The drawing under review shows one solid part. Ordinate dimensions are in mm from its lowest x, y, z. A direction names the side the tool comes from. Round coordinates to 2 decimals unless told otherwise and drop trailing zeros. Loops run counter-clockwise (first coordinate to the right, second up) from the corner with the lowest first, then second, coordinate; pieces in that order, holes last. Notation, with made-up numbers: (52.25, 3.5) - (100.25, 3.5) arc R26 cw to (100.25, 19.5) - close; hole circle Ø9 at (-16, 55). An arc over 180 degrees is marked (long way). Answer as CSV lines item,"result".
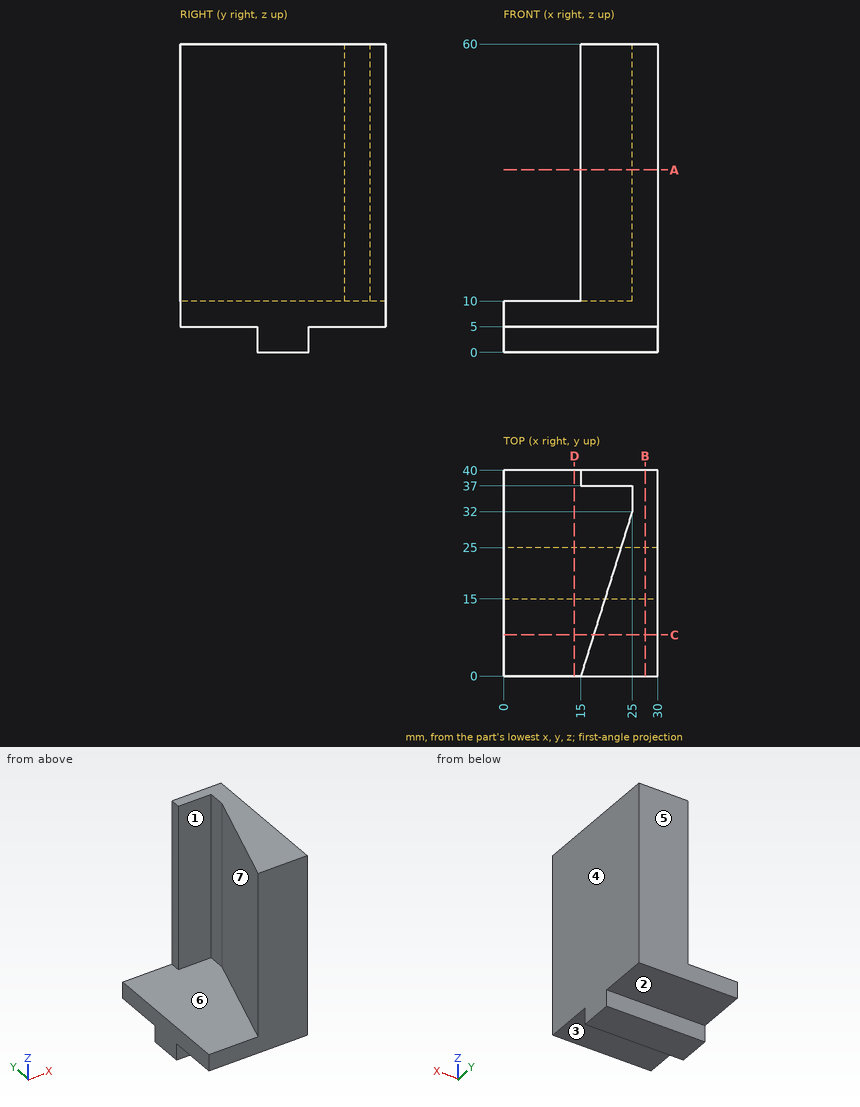
1. Take a section at D-D (x = 13.75). State the section outline as (y, z) points.
Numbers:
outline,"(0, 5) - (15, 5) - (15, 0) - (25, 0) - (25, 5) - (40, 5) - (40, 10) - (0, 10) - close"
2. Tool access review of the marked faces 1, 2 and 3: name each direction out of +Z, -Z, +X, -X, +Y, -Y from which nothing blocks a thin tool from reaching the whole face with its end or side.
Numbers:
face 1,"+Z, -X"
face 2,"-Z, +X, -X, +Y"
face 3,"-Z, +X, -X, -Y"
3. Wall thickness on probe 1 along Z at (x, y) = (9.25, 13); probe 2 along Z at (x, y) = (7.75, 24.5); probe 3 along Y at (x, z) = (4.75, 3.5): over which ranges is each line inside the solid? List them lowest first.
Numbers:
probe 1,"z = 5 to 10"
probe 2,"z = 0 to 10"
probe 3,"y = 15 to 25"
4. Draft analysis for pull direction Y (two halves, no side actions). For the marked faces 4, 5, 6 and 7, state which applies: +Y half, -Y half, draft (parallel to the pull), parting line (faces both ways), or undercut.
Numbers:
face 4,"draft"
face 5,"+Y half"
face 6,"undercut"
face 7,"undercut"
5. Take a section at C-C (y = 8). State the section outline as (x, z) points, plus the area to 3 significant figures.
Numbers:
outline,"(0, 5) - (30, 5) - (30, 60) - (17.5, 60) - (17.5, 10) - (0, 10) - close"
area,"775 mm²"
6. Clearance check with flat-ended pins moving along their axes: pin 1 (1 mm diameter, centred on x = 6, y = 33.5, fed in from +Z); pin 2 (1.5 mm diameter, centred on y = 24, z = 36.5, fed in from -X); pin 3 (5.5 mm diameter, centred on y = 35.5, z = 24, fed in from -X). State where each tip first meets the part, or that it passes through.
Numbers:
pin 1,"stops at z = 10"
pin 2,"stops at x = 22.27"
pin 3,"stops at x = 15"
7. Take a section at A-A (z = 35.5). State the section outline as (x, y) points.
Numbers:
outline,"(15, 0) - (30, 0) - (30, 40) - (15, 40) - (15, 37) - (25, 37) - (25, 32) - close"
8. Take a section at B-B (x = 27.5). State the section outline as (y, z) points.
Numbers:
outline,"(0, 5) - (15, 5) - (15, 0) - (25, 0) - (25, 5) - (40, 5) - (40, 60) - (0, 60) - close"
